Can you work these out from the model? Positions are in its coordinate system, mm. A direction names the side the tool comes from. Round coordinates to 2 decimals unless told otherwise and drop trailing zeros. Write each loop counter-clockwise with the first axis right and the second up, starting at its lowest first coordinate (ties: lowest second). Pieces come first, ordered by that corner, then holes. Notation, with made-up numbers: (-27, 74) -> (-17, 74) arc R10 cw to (-17, 91) -> close; hole circle Ø5 at (38, 80.25). An arc over 180 degrees is marked (long way). Use CSV: the item, a comma, the result in double quotes.
```python
from build123d import *

# Parameters (mm, degrees)
F0_R      = 4.7625
F1_DEPTH  = 12.7
F2_R      = 6.35
F3_R      = 3.175
F4_R      = 1.8415
F5_DEPTH  = 25.4
F7_DEPTH  = 3.175
F8_R      = 1.8415
F9_DEPTH  = 25.4
F11_DEPTH = 3.175


with BuildPart() as f1:
    # F0 (on Top) → F1 (new body)
    with BuildSketch(Plane.XY):
        Polygon((-13.335, 18.415), (-13.335, -13.335), (18.415, -13.335), (18.415, -6.985), (7.62, -6.985), (7.62, 7.62), (-6.985, 7.62), (-6.985, 18.415), align=None)
        Circle(F0_R, mode=Mode.SUBTRACT)
    extrude(amount=F1_DEPTH)

    # F2
    f2_edges = [f1.edges().sort_by_distance(p)[0] for p in [
        (7.62, 7.62, 6.35),
    ]]
    fillet(f2_edges, radius=F2_R)

    # F3
    f3_edges = [f1.edges().sort_by_distance(p)[0] for p in [
        (-13.335, -13.335, 6.35),
    ]]
    fillet(f3_edges, radius=F3_R)

    # F4 (on face) → F5 (cut)
    with BuildSketch(Plane(origin=(0, -6.985, 0), x_dir=(-1, 0, 0), z_dir=(0, 1, 0))):
        with Locations((-13.0175, 6.35)):
            Circle(F4_R)
    extrude(amount=-F5_DEPTH, mode=Mode.SUBTRACT)

    # F6 (on face) → F7 (cut)
    with BuildSketch(Plane(origin=(0, -6.985, 0), x_dir=(-1, 0, 0), z_dir=(0, 1, 0))):
        Polygon((-17.0815, 4.003649), (-13.0175, 1.657297), (-8.9535, 4.003649), (-8.9535, 8.696351), (-13.0175, 11.042703), (-17.0815, 8.696351), align=None)
    extrude(amount=-F7_DEPTH, mode=Mode.SUBTRACT)

    # F8 (on face) → F9 (cut)
    with BuildSketch(Plane.YZ.offset(-6.985)):
        with Locations((13.0175, 6.35)):
            Circle(F8_R)
    extrude(amount=-F9_DEPTH, mode=Mode.SUBTRACT)

    # F10 (on face) → F11 (cut)
    with BuildSketch(Plane.YZ.offset(-6.985)):
        Polygon((8.9535, 8.696351), (8.9535, 4.003649), (13.0175, 1.657297), (17.0815, 4.003649), (17.0815, 8.696351), (13.0175, 11.042703), align=None)
    extrude(amount=-F11_DEPTH, mode=Mode.SUBTRACT)


solid = f1.part
```
Q1. If we mould it in two halves opening along Y, with no side actions, what happens to faces 5 (the face through (-8.55, 15.08, 9.85)), 6 (the face through (12, -6.985, 2)), 7 (the face through (-9, 8.954, 6)), 8 (the face through (-6.985, 14, 2))? For each: released by +Y, released by -Y, zero draft, split by the parting line, or undercut.
Resolved:
face 5,"undercut"
face 6,"released by +Y"
face 7,"undercut"
face 8,"zero draft"
Q2. Please list where these lines run through material, in increasing order: probe 1 along X at (y, z) = (14, 8.75) (3 decimals); probe 2 along X at (y, z) = (-12, 6.5) (3 decimals); probe 3 along X at (y, z) = (15, 2) (3 decimals).
Resolved:
probe 1,"x = -13.335 to -10.16"
probe 2,"x = -12.747 to 11.182, 14.853 to 18.415"
probe 3,"x = -13.335 to -6.985"
Q3. On a 3-axis mill with a long thin cutter (end or side, diameter ignored), from which of +Z, -Z, +X, -X, +Y, -Y can I reach the whole of each face in a straight line? I mean faces 1 (the face through (4, -13.335, 6)), 2 (the face through (-8.55, 11.014, 9.886)), 3 (the face through (7.62, -3, 6)), 4 (the face through (10.957, -8.55, 9.853)). Say none if no direction works.
Resolved:
face 1,"+Z, -Z, +X, -X, -Y"
face 2,"+X"
face 3,"+Z, -Z, +X, +Y"
face 4,"+Y"
Q4. Suppose I cut it at B-B (y = 0). Write out the boundary of the cut face in (x, z) (1 decimal).
Resolved:
outline,"(-13.3, 0) -> (-4.8, 0) -> (-4.8, 12.7) -> (-13.3, 12.7) -> close; (4.8, 0) -> (7.6, 0) -> (7.6, 12.7) -> (4.8, 12.7) -> close"
Q5. Suppose I cut it at A-A (z = 6.35). Count the separate pieces of the cut face and the enclosed holes in it, and give its area (3 significant figures).
Resolved:
separate pieces,"3"
enclosed holes,"1"
area,"419 mm^2"
Q6. Will these pins go through, and if not, where does the flat tip stop? P1, Ø1.5, axis at y = 4.5, z = 4.5, coming from the +X side; P2, Ø4, axis at x = 11.5, z = 8, coming from the +Y side (3 decimals); P3, Ø2.5, axis at y = -2, z = 6.5, coming from the +X side.
Resolved:
P1,"stops at x = 7.12"
P2,"stops at y = -6.985"
P3,"stops at x = 7.62"
